from build123d import *

# Parameters (mm, degrees)
SKETCH1_W           = 9.525
SKETCH1_H           = 16.6624
BOSS_EXTRUDE1_DEPTH = 0.8128
SKETCH2_W           = 9.525
SKETCH2_H           = 0.8128
BOSS_EXTRUDE2_DEPTH = 28.5496
SKETCH3_R           = 2.1463
CUT_EXTRUDE1_DEPTH  = 35.401175255
SKETCH4_R           = 2.1463
CUT_EXTRUDE2_DEPTH  = 35.699942059


with BuildPart() as part:
    # Sketch1 → Boss-Extrude1 (new body)
    with BuildSketch(Plane(origin=(0, 0, 0), x_dir=(1, 0, 0), z_dir=(0, 1, 0))):
        with Locations((4.7625, 8.3312)):
            Rectangle(SKETCH1_W, SKETCH1_H)
    extrude(amount=BOSS_EXTRUDE1_DEPTH)

    # Sketch2 → Boss-Extrude2 (add)
    with BuildSketch(Plane(origin=(0, 0.8128, 0), x_dir=(1, 0, 0), z_dir=(0, 1, 0))):
        with Locations((4.7625, 16.256)):
            Rectangle(SKETCH2_W, SKETCH2_H)
    extrude(amount=BOSS_EXTRUDE2_DEPTH)

    # Sketch3 → Cut-Extrude1 (cut, through all)
    with BuildSketch(Plane(origin=(0, 0.8128, 0), x_dir=(1, 0, 0), z_dir=(0, 1, 0))):
        with Locations(Location((4.7625, 6.35, 0), (0, 0, 270))):
            Circle(SKETCH3_R)
    extrude(amount=-CUT_EXTRUDE1_DEPTH, mode=Mode.SUBTRACT)

    # Sketch4 → Cut-Extrude2 (cut, through all)
    with BuildSketch(Plane.XY.offset(-15.8496)):
        with Locations((4.7625, 23.0124)):
            Circle(SKETCH4_R)
    extrude(amount=-CUT_EXTRUDE2_DEPTH, mode=Mode.SUBTRACT)


solid = part.part
The listing builds one solid part. Answer for the finished solid, in the listing's coordinates (mm). A direction names the side the tool comes from. Coordinates: 2 decimals unless noted, no trailing zeros. Loops run counter-clockwise (first coordinate to the right, second up) from the corner with the lowest first, then second, coordinate; pieces in that order, holes last.
1) Find section C-C on x = 2. Write down the section's boundary in (y, z), then the cut area to 3 significant figures.
2) A tool of negligible diameter and unlimited length cuts with its end or side. For faces 4 (the face through (2.86, 0.41, -5.36)), 5 (the face through (5, 15, -15.85)), from which of +Z, -Z, +X, -X, +Y, -Y can it reach the whole face along a straight path? Write none if from no direction.
3) Find section B-B on y = 24.75. Write down the section's boundary in (x, z) (3 decimals), then the cut area to 3 significant figures.
4) Determine the mould class of faces 1 (the face through (5, 0.813, -10)), 2 (the face through (5.92, 24.82, -16.25)), 3 (the face through (4.7, 0.4, 0)) for opening direction Y: pulls with the +Y half, pulls with the -Y half, needs draft (parallel to the pull), parting line crosses it, or undercut.
5) Find section D-D on y = 4.25. Write down the section's boundary in (x, z) (3 decimals), then the cut area to 3 significant figures.
6) Find section A-A on z = -6.35. Write down the section's boundary in (x, y) (3 decimals).
7) Find the intervals of material crossed by L1, parallel to Y at x = 7, z = -12.25; L2, parallel to Z at x = 2.75, y = 22, in increasing order.
8) Flat-ended cylindrical pins translate along their axes: pin 1 Ø5 at (x, y) = (4.76, 23.01) entering from +Z; pin 2 Ø5 at (x, z) = (6.5, -12) entering from +Y. Find the tip coordinate at first contact, or state that the pin passes through.
Values:
1. outline: (0, -16.66) - (29.36, -16.66) - (29.36, -15.85) - (0.81, -15.85) - (0.81, 0) - (0, 0) - close
1. area: 36.7 mm2
2. face 4: +Y, -Y
2. face 5: +Z, +X, -X, +Y
3. outline: (0, -16.662) - (3.503, -16.662) - (3.503, -15.85) - (0, -15.85) - close; (6.022, -16.662) - (9.525, -16.662) - (9.525, -15.85) - (6.022, -15.85) - close
3. area: 5.69 mm2
4. face 1: pulls with the +Y half
4. face 2: undercut
4. face 3: needs draft
5. outline: (0, -16.662) - (9.525, -16.662) - (9.525, -15.85) - (0, -15.85) - close
5. area: 7.74 mm2
6. outline: (0, 0) - (2.616, 0) - (2.616, 0.813) - (0, 0.813) - close; (6.909, 0) - (9.525, 0) - (9.525, 0.813) - (6.909, 0.813) - close
7. L1: y = 0 to 0.81
7. L2: z = -16.66 to -15.85
8. pin 1: stops at z = -15.85
8. pin 2: stops at y = 0.81
